```python
from build123d import *

# Parameters (mm, degrees)
SKETCH_1_W             = 117.567875581
SKETCH_1_H             = 35.211732604
EXTRUDE_1_DEPTH        = 2
SKETCH_3_W             = 0.8
SKETCH_3_H             = 1.2
SKETCH_3_W_2           = 1
SKETCH_3_H_2           = 0.8
CUT_EXTRUDE_1_DEPTH    = 123.743926455
PATTERN_LINEAR_1_COUNT = 3
PATTERN_LINEAR_1_PITCH = 20
SKETCH_4_OUTSIDE_W     = 144.116
SKETCH_4_OUTSIDE_H     = 61.76
SKETCH_4_OUTSIDE_W_2   = 50
SKETCH_4_OUTSIDE_H_2   = 6.9
CUT_EXTRUDE_2_DEPTH    = 123.743926455
SKETCH_5_W             = 6.2
SKETCH_5_H             = 2.8
SKETCH_5_W_2           = 6
EXTRUDE_2_DEPTH        = 7
SKETCH_6_R             = 2
CUT_EXTRUDE_3_DEPTH    = 1.5
SKETCH_6_3_R           = 1
CUT_EXTRUDE_4_DEPTH    = 51.653825127


with BuildPart() as part:
    # 草图1 → 凸台-拉伸1 (new body)
    with BuildSketch(Plane(origin=(0, 0, 0), x_dir=(1, 0, 0), z_dir=(0, 1, 0))):
        with Locations((58.783937791, -17.605866302)):
            Rectangle(SKETCH_1_W, SKETCH_1_H)
    extrude(amount=EXTRUDE_1_DEPTH)

    # 草图3 → 切除-拉伸1 (cut, through all)
    with BuildSketch(Plane(origin=(0, 2, 0), x_dir=(1, 0, 0), z_dir=(0, 1, 0))):
        with Locations((1.5, -5.4)):
            Rectangle(SKETCH_3_W, SKETCH_3_H)
        with Locations((8.5, -5.4)):
            Rectangle(SKETCH_3_W, SKETCH_3_H)
        with Locations((2.8, -3)):
            Rectangle(SKETCH_3_W_2, SKETCH_3_H_2)
        with Locations((7.2, -3)):
            Rectangle(SKETCH_3_W_2, SKETCH_3_H_2)
    cut_extrude_1 = extrude(amount=-CUT_EXTRUDE_1_DEPTH, mode=Mode.SUBTRACT)

    # 阵列(线性)1: 切除-拉伸1 ×3
    with Locations(*[(i * PATTERN_LINEAR_1_PITCH, 0, 0) for i in range(1, PATTERN_LINEAR_1_COUNT)]):
        add(cut_extrude_1, mode=Mode.SUBTRACT)

    # 草图4 outside → 切除-拉伸2 (cut, through all)
    with BuildSketch(Plane.XZ):
        with Locations((58.784, 17.606)):
            Rectangle(SKETCH_4_OUTSIDE_W, SKETCH_4_OUTSIDE_H)
        with Locations((25, 3.45)):
            Rectangle(SKETCH_4_OUTSIDE_W_2, SKETCH_4_OUTSIDE_H_2, mode=Mode.SUBTRACT)
    extrude(amount=-CUT_EXTRUDE_2_DEPTH, mode=Mode.SUBTRACT)

    # 草图5 → 凸台-拉伸2 (add)
    with BuildSketch(Plane.XZ):
        with Locations((45, 5.5)):
            Rectangle(SKETCH_5_W, SKETCH_5_H)
        with Locations((25, 5.5)):
            Rectangle(SKETCH_5_W, SKETCH_5_H)
        with Locations((5, 5.5)):
            Rectangle(SKETCH_5_W, SKETCH_5_H)
        with Locations((15, 5.5)):
            Rectangle(SKETCH_5_W_2, SKETCH_5_H)
        with Locations((35, 5.5)):
            Rectangle(SKETCH_5_W_2, SKETCH_5_H)
    extrude(amount=EXTRUDE_2_DEPTH)

    # 草图6 → 切除-拉伸3 (cut)
    with BuildSketch(Plane(origin=(0, 0, 4.1), x_dir=(-1, 0, 0), z_dir=(0, 0, -1))):
        with Locations((-35, -3.5)):
            Circle(SKETCH_6_R)
        with Locations((-15, -3.5)):
            Circle(SKETCH_6_R)
    extrude(amount=-CUT_EXTRUDE_3_DEPTH, mode=Mode.SUBTRACT)

    # 草图6<3> → 切除-拉伸4 (cut, through all)
    with BuildSketch(Plane(origin=(0, 0, 4.1), x_dir=(-1, 0, 0), z_dir=(0, 0, -1))):
        with Locations((-35, -3.5)):
            Circle(SKETCH_6_3_R)
        with Locations((-15, -3.5)):
            Circle(SKETCH_6_3_R)
    extrude(amount=-CUT_EXTRUDE_4_DEPTH, mode=Mode.SUBTRACT)


solid = part.part
```
Check sheet for the modelled part. Datum: model origin and axes. Units: mm. A direction names the side the tool comes from. Give positions to 0.01 mm unless a question says otherwise; leave off trailing zeros. Order: outer loops, then holes, each group sorted by start corner. A loop starts at its lowest first (then second) coordinate and runs counter-clockwise, first axis right, second up. Notation, with made-up numbers: M -18,17.5 L 35,17.5 A20 ccw 35,50.5 Z; hole C -8.5,56 d7. An arc over 180 degrees is marked long. Answer in a Markdown table with one row per item.
1) Cross-section at D-D, the plane y = -3.5. Count the separate pieces of the cut face and the enclosed holes in it, plus the area to 3 significant figures.
Filled sheet:
| item | result |
|---|---|
| separate pieces | 7 |
| enclosed holes | 0 |
| area | 68.5 mm2 |
2) Release check for a two-part mould opening along Y. For faces 4 (the cylindrical face through (16.6, -4.7, 4.8)), 5 (the flat face through (25, -7, 6)), 6 (the flat face through (14.1, -4.4, 5.6)), 7 (the flat face through (21.1, 1, 5)) record: +Y half, -Y half, draft (parallel to the pull), parting line (faces both ways), or undercut.
Filled sheet:
| item | result |
|---|---|
| face 4 | undercut |
| face 5 | -Y half |
| face 6 | undercut |
| face 7 | draft |
3) Thickness scan on L1, parallel to Y at x = 15, z = 6; L2, parallel to Y at x = 15, z = 4.55; L3, parallel to Y at x = 31.5, z = 2. Record the ranges inside material, lowest first. Write a range as [from, to].
Filled sheet:
| item | result |
|---|---|
| L1 | y = [-7, -4.5], [-2.5, 2] |
| L2 | y = [-7, -5.5], [-1.5, 2] |
| L3 | y = [0, 2] |
4) Cross-section at C-C, the plane x = 6. Enter the section's corners in (y, z), plus the area to 3 significant figures.
Filled sheet:
| item | result |
|---|---|
| outline | M -7,4.1 L 0,4.1 L 0,0 L 2,0 L 2,6.9 L -7,6.9 Z |
| area | 33.4 mm2 |
5) Access from +Z, -Z, +X, -X, +Y, -Y to the whole of each face (thin tool, end or side, straight path). Record for faces 1 (the flat face through (5, -3, 4.1)), 2 (the flat face through (26.7, 1, 3)), 3 (the flat face through (50, 1, 3)).
Filled sheet:
| item | result |
|---|---|
| face 1 | -Z, +X, -X, -Y |
| face 2 | +Y, -Y |
| face 3 | +Z, -Z, +X, +Y, -Y |
6) Cross-section at B-B, the plane x = 15. Enter the section's corners in (y, z).
Filled sheet:
| item | result |
|---|---|
| outline | M -7,4.1 L -5.5,4.1 L -5.5,5.6 L -4.5,5.6 L -4.5,6.9 L -7,6.9 Z; M -2.5,5.6 L -1.5,5.6 L -1.5,4.1 L 0,4.1 L 0,0 L 2,0 L 2,6.9 L -2.5,6.9 Z |
7) Cross-section at A-A, the plane y = -1. Enter the section's corners in (x, z).
Filled sheet:
| item | result |
|---|---|
| outline | M 1.9,4.1 L 8.1,4.1 L 8.1,6.9 L 1.9,6.9 Z; M 12,4.1 L 18,4.1 L 18,6.9 L 12,6.9 Z; M 21.9,4.1 L 28.1,4.1 L 28.1,6.9 L 21.9,6.9 Z; M 32,4.1 L 38,4.1 L 38,6.9 L 32,6.9 Z; M 41.9,4.1 L 48.1,4.1 L 48.1,6.9 L 41.9,6.9 Z |
8) Gauge pin test, flat ends, axial feed: P1, Ø4, axis at y = -2.5, z = 5, coming from the -X side; P2, Ø2, axis at x = 15.5, y = -5, coming from the -Z side; P3, Ø2, axis at y = -4, z = 6, coming from the +X side. Record the tip position at first contact, or that the pin passes through.
Filled sheet:
| item | result |
|---|---|
| P1 | stops at x = 1.9 |
| P2 | stops at z = 4.1 |
| P3 | stops at x = 48.1 |
